from build123d import *

# Parameters (mm, degrees)
SKETCH1_R           = 2
SKETCH1_R_2         = 11.5
SKETCH1_R_3         = 4.5
SKETCH1_R_4         = 1.5
BOSS_EXTRUDE1_DEPTH = 10


with BuildPart() as part:
    # Sketch1 → Boss-Extrude1 (new body)
    with BuildSketch(Plane.XY):
        with BuildLine():
            Line((0, 0), (360, 0))
            Line((360, 0), (360, -45))
            Line((360, -45), (340, -45))
            Line((340, -45), (340, -40))
            ThreePointArc((340, -40), (339.121320344, -37.878679656), (337, -37))
            Line((337, -37), (23, -37))
            ThreePointArc((23, -37), (20.878679656, -37.878679656), (20, -40))
            Line((20, -40), (20, -45))
            Line((20, -45), (0, -45))
            Line((0, -45), (0, 0))
        make_face()
        with Locations((350, -10)):
            Circle(SKETCH1_R, mode=Mode.SUBTRACT)
        with Locations((350, -30)):
            Circle(SKETCH1_R, mode=Mode.SUBTRACT)
        with Locations((10, -10)):
            Circle(SKETCH1_R, mode=Mode.SUBTRACT)
        with Locations((10, -30.004476127)):
            Circle(SKETCH1_R, mode=Mode.SUBTRACT)
        with Locations((180, -18.5)):
            Circle(SKETCH1_R_2, mode=Mode.SUBTRACT)
        with Locations((255, -18.5)):
            Circle(SKETCH1_R_3, mode=Mode.SUBTRACT)
        with Locations((105, -18.5)):
            Circle(SKETCH1_R_3, mode=Mode.SUBTRACT)
        with Locations((164, -5)):
            Circle(SKETCH1_R_4, mode=Mode.SUBTRACT)
        with Locations((196, -5)):
            Circle(SKETCH1_R_4, mode=Mode.SUBTRACT)
        with Locations((196, -32)):
            Circle(SKETCH1_R_4, mode=Mode.SUBTRACT)
        with Locations((164, -32)):
            Circle(SKETCH1_R_4, mode=Mode.SUBTRACT)
    extrude(amount=BOSS_EXTRUDE1_DEPTH)


solid = part.part
The listing builds one solid part. Answer for the finished solid, in the listing's coordinates (mm). A direction names the side the tool comes from. Coordinates: 2 decimals unless noted, no trailing zeros. Order: outer loops, then holes, each group sorted by start corner. A loop starts at its lowest first (then second) coordinate and runs counter-clockwise, first axis right, second up.
Q1. Which of the six approach directions +Z, -Z, +X, -X, +Y, -Y give full straight-line access (tool end or side, diameter ignored) to faces 4 (the face through (182, -37, 5)), 5 (the face through (259.292, -17.148, 4.93))?
Q2. A cutting plane is placed at B-B, the plane y = -18.5. Write down the section's boundary in (x, z), and give its area (3 significant figures).
Q3. A cutting plane is placed at D-D, the plane x = 105. Write down the section's boundary in (y, z).
Q4. Given P1, Ø3, axis at y = -23, z = 3.5, coming from the -X side; P2, Ø2, axis at x = 245, z = 3.5, coming from the -Y side, each flat-ended and moving along its own axis, determine where each tip first touches the part or whether it passes through.
Q5. For a pull along Y with two mould halves and no side action, classify faces 1 (the face through (100.504, -18.302, 4.93)), 2 (the face through (183, -7, 10)), 3 (the face through (10, -45, 5)) as pulls with the +Y half, pulls with the -Y half, needs draft (parallel to the pull), parting line crosses it, or undercut.
Q6. Consider line 1 (X direction, y = -41, z = 8.75); line 2 (X direction, y = -28.5, z = 1.5); line 3 (Y direction, x = 255, z = 4.25). Determine where each line is inside the solid, lowest interval first.
Q7. A cutting plane is placed at A-A, the plane x = 180. Write down the section's boundary in (y, z), and give its area (3 significant figures).
Q8. A cutting plane is placed at C-C, the plane z = 3.5. State how many separate pieces and enclosed holes the cut face has, and give its area (3 significant figures).
Answers follow:
1. face 4: +Z, -Z, -Y
1. face 5: +Z, -Z
2. outline: (0, 0) - (100.5, 0) - (100.5, 10) - (0, 10) - close; (109.5, 0) - (168.5, 0) - (168.5, 10) - (109.5, 10) - close; (191.5, 0) - (250.5, 0) - (250.5, 10) - (191.5, 10) - close; (259.5, 0) - (360, 0) - (360, 10) - (259.5, 10) - close
2. area: 3,190 mm2
3. outline: (-37, 0) - (-23, 0) - (-23, 10) - (-37, 10) - close; (-14, 0) - (0, 0) - (0, 10) - (-14, 10) - close
4. P1: stops at x = 0
4. P2: stops at y = -37
5. face 1: undercut
5. face 2: needs draft
5. face 3: pulls with the -Y half
6. line 1: x = 0 to 20, 340 to 360
6. line 2: x = 0 to 8.68, 11.32 to 174.32, 185.68 to 348.68, 351.32 to 360
6. line 3: y = -37 to -23, -14 to 0
7. outline: (-37, 0) - (-30, 0) - (-30, 10) - (-37, 10) - close; (-7, 0) - (0, 0) - (0, 10) - (-7, 10) - close
7. area: 140 mm2
8. separate pieces: 1
8. enclosed holes: 11
8. area: 13,000 mm2
